The model under review builds one solid part; all positions refer to its coordinate system, in mm. A direction names the side the tool comes from. Coordinates: 2 decimals unless noted, no trailing zeros. Loops run counter-clockwise (first coordinate to the right, second up) from the corner with the lowest first, then second, coordinate; pieces in that order, holes last. Notation, with made-up numbers: M 78.5,-15.5 L 87.5,-15.5 A18 ccw 87.5,-3.5 Z; hole C -6.75,71.25 d1. An arc over 180 degrees is marked long. Return JSON: item names as keys, results as strings.
```python
from build123d import *

# Parameters (mm, degrees)
F0_W     = 69.795026
F0_H     = 78.517704
F1_DEPTH = 16.002
F3_DEPTH = 13.462


with BuildPart() as f1:
    # F0 (on Right) → F1 (new body)
    with BuildSketch(Plane.YZ):
        with Locations((-1.721126, 11.479196)):
            Rectangle(F0_W, F0_H)
    extrude(amount=F1_DEPTH)

    # F2 (on face) → F3 (join)
    with BuildSketch(Plane.YZ.offset(16.002)):
        Polygon((0, 14.234204), (0, 50.738048), (-36.618639, 50.738048), (-36.618639, -11.249613), (33.176387, -11.249613), (33.176387, 14.234204), align=None)
    extrude(amount=F3_DEPTH)


solid = f1.part
```
1. To check wall thickness, follow line 1 (X direction, y = 18, z = 27.5); line 2 (Z direction, x = 26.25, y = 7); line 3 (Y direction, x = 17.5, z = 40). State the ranges of each line that lie inside material, in increasing order.
Check values:
{"line 1": "0 to 16", "line 2": "-11.25 to 14.23", "line 3": "-36.62 to 0"}
2. Add section B-B on z = 39.5. Give the boundary of the cut face in (x, y), plus the area to 3 significant figures.
Check values:
{"outline": "M 0,-36.62 L 29.46,-36.62 L 29.46,0 L 16,0 L 16,33.18 L 0,33.18 Z", "area": "1,610 mm²"}
3. Add section A-A on y = 26. Give the boundary of the cut face in (x, z).
Check values:
{"outline": "M 0,-27.78 L 16,-27.78 L 16,-11.25 L 29.46,-11.25 L 29.46,14.23 L 16,14.23 L 16,50.74 L 0,50.74 Z"}
4. Add section D-D on z = -14. Give the boundary of the cut face in (x, y).
Check values:
{"outline": "M 0,-36.62 L 16,-36.62 L 16,33.18 L 0,33.18 Z"}
5. Machinability: for faces 1 (the face through (16.002, -2, -19)), 2 (the face through (23, 17, 14.234)), 3 (the face through (15, -36.619, 12)), which of the approach directions +Z, -Z, +X, -X, +Y, -Y give a long, thin tool a straight path to every point of the face, cutting with its end or side? Answer none if there is none.
Check values:
{"face 1": "-Z, +X, +Y, -Y", "face 2": "+Z, +X, +Y", "face 3": "+Z, -Z, +X, -X, -Y"}
6. Insertion check: pin 1 Ø2 at (x, z) = (24, 37.5) entering from +Y; pin 2 Ø8.5 at (y, z) = (-6.5, -20) entering from +X; pin 3 Ø6.5 at (x, y) = (23.5, 3) entering from -Z. Each pin has a flat end and moves straight along its axis. Give the tip position at first contact, or say it passes through.
Check values:
{"pin 1": "y = 0", "pin 2": "x = 16", "pin 3": "z = -11.25"}
7. Add section C-C on x = 17.5. Give the boundary of the cut face in (y, z).
Check values:
{"outline": "M -36.62,-11.25 L 33.18,-11.25 L 33.18,14.23 L 0,14.23 L 0,50.74 L -36.62,50.74 Z"}
